Can you work these out from the model? Positions are in its coordinate system, mm. A direction names the side the tool comes from. Round coordinates to 2 decimals unless told otherwise and drop trailing zeros. Write each loop counter-clockwise with the first axis right and the second up, starting at its lowest first coordinate (ties: lowest second). Pieces come first, ordered by that corner, then holes. Notation, with made-up numbers: (64.25, -25) -> (114.25, -25) arc R25 ccw to (114.25, -6) -> close; hole circle Ø8 at (15, -10). An arc over 180 degrees is marked (long way). Use CSV: the item, a comma, the result in double quotes.
```python
from build123d import *

# Parameters (mm, degrees)
F0_W     = 35.12067
F0_H     = 33.25997
F0_R     = 8.477478
F1_DEPTH = 101.6
F2_R     = 45.532987
F3_DEPTH = 50.8
F4_R     = 7.387342
F5_DEPTH = 254


with BuildPart() as f1:
    # F0 (on Front) → F1 (new body)
    with BuildSketch(Plane.XZ):
        Rectangle(F0_W, F0_H)
        Circle(F0_R, mode=Mode.SUBTRACT)
    extrude(amount=F1_DEPTH)

    # F2 (on Front) → F3 (join)
    with BuildSketch(Plane.XZ):
        Circle(F2_R)
    extrude(amount=F3_DEPTH)

    # F4 (on Front) → F5 (join)
    with BuildSketch(Plane.XZ):
        Circle(F4_R)
    extrude(amount=F5_DEPTH)


solid = f1.part
```
Q1. Please list where these lines run through material, in increasing order: probe 1 along Z at (x, y) = (0, -70); probe 2 along X at (y, z) = (-71, 0); probe 3 along Y at (x, z) = (12.5, 36).
Resolved:
probe 1,"z = -16.63 to -8.48, -7.39 to 7.39, 8.48 to 16.63"
probe 2,"x = -17.56 to -8.48, -7.39 to 7.39, 8.48 to 17.56"
probe 3,"y = -50.8 to 0"
Q2. Suppose I cut it at A-A (y = -98). Write out the boundary of the cut face in (x, z), and give its area (3 significant figures).
Resolved:
outline,"(-17.56, -16.63) -> (17.56, -16.63) -> (17.56, 16.63) -> (-17.56, 16.63) -> close; circle Ø14.77 at (0, 0); hole circle Ø16.95 at (0, 0)"
area,"1,110 mm^2"
Q3. On a 3-axis mill with a long thin cutter (end or side, diameter ignored), from which of +Z, -Z, +X, -X, +Y, -Y can I reach the whole of each face in a straight line? I mean faces 1 (the face through (0, -76, 16.63)), 2 (the face through (-17.56, -76, 0)), 3 (the face through (-5.86, -150.98, -4.5)), 4 (the face through (17.56, -76, 0)), 5 (the face through (0, -76, -16.63)). Say none if no direction works.
Resolved:
face 1,"+Z, +X, -X, -Y"
face 2,"+Z, -Z, -X, -Y"
face 3,"-Y"
face 4,"+Z, -Z, +X, -Y"
face 5,"-Z, +X, -X, -Y"
Q4. Suppose I cut it at D-D (y = -157). Write out the boundary of the cut face in (x, z), and give its area (3 significant figures).
Resolved:
outline,"circle Ø14.77 at (0, 0)"
area,"171 mm^2"
Q5. If we mould it in two halves opening along X, with no side actions, what happens to faces 6 (the face through (7.83, -75.84, -3.25)), 7 (the face through (-1, 0, 1)), 8 (the face through (43.43, -25.04, 13.68))? For each: released by +X, released by -X, zero draft, split by the parting line, or undercut.
Resolved:
face 6,"undercut"
face 7,"zero draft"
face 8,"split by the parting line"
Q6. Suppose I cut it at C-C (z = 0). Write out the boundary of the cut face in (x, y), and give its area (3 significant figures).
Resolved:
outline,"(-45.53, -50.8) -> (-17.56, -50.8) -> (-17.56, -101.6) -> (-8.48, -101.6) -> (-8.48, -50.8) -> (-7.39, -50.8) -> (-7.39, -254) -> (7.39, -254) -> (7.39, -50.8) -> (8.48, -50.8) -> (8.48, -101.6) -> (17.56, -101.6) -> (17.56, -50.8) -> (45.53, -50.8) -> (45.53, 0) -> (-45.53, 0) -> close"
area,"8,550 mm^2"
Q7. Suppose I cut it at B-B (x = 0). Write out the boundary of the cut face in (y, z).
Resolved:
outline,"(-254, -7.39) -> (-50.8, -7.39) -> (-50.8, -8.48) -> (-101.6, -8.48) -> (-101.6, -16.63) -> (-50.8, -16.63) -> (-50.8, -45.53) -> (0, -45.53) -> (0, 45.53) -> (-50.8, 45.53) -> (-50.8, 16.63) -> (-101.6, 16.63) -> (-101.6, 8.48) -> (-50.8, 8.48) -> (-50.8, 7.39) -> (-254, 7.39) -> close"
Q8. Will these pins go through, and if not, where does the flat tip stop? P1, Ø1, axis at x = -19.5, z = -11.5, coming from the -Y side; P2, Ø3, axis at x = 15, y = -40.5, coming from the +Z side; P3, Ø16.5, axis at y = -87, z = 6, coming from the -X side.
Resolved:
P1,"stops at y = -50.8"
P2,"stops at z = 43.49"
P3,"stops at x = -17.56"
